from build123d import *

# Parameters (mm, degrees)
BOSS_EXTRUDE1_DEPTH = 3.175


with BuildPart() as part:
    # Sketch1 → Boss-Extrude1 (new body)
    with BuildSketch(Plane(origin=(0, 0, 0), x_dir=(1, 0, 0), z_dir=(0, 1, 0))):
        Polygon((0, -25.4), (0, 25.4), (25.4, 25.4), (25.4, 28.575), (114.3, 28.575), (114.3, 25.4), (139.7, 25.4), (165.1, 25.4), (165.1, 28.575), (254, 28.575), (254, 25.4), (279.4, 25.4), (304.8, 25.4), (304.8, 28.575), (393.7, 28.575), (393.7, 25.4), (419.1, 25.4), (444.5, 25.4), (444.5, 28.575), (533.4, 28.575), (533.4, 25.4), (558.8, 25.4), (558.8, -25.4), (533.4, -25.4), (533.4, -28.575), (444.5, -28.575), (444.5, -25.4), (419.1, -25.4), (393.7, -25.4), (393.7, -28.575), (304.8, -28.575), (304.8, -25.4), (279.4, -25.4), (254, -25.4), (254, -28.575), (165.1, -28.575), (165.1, -25.4), (139.7, -25.4), (114.3, -25.4), (114.3, -28.575), (25.4, -28.575), (25.4, -25.4), align=None)
    extrude(amount=BOSS_EXTRUDE1_DEPTH)


solid = part.part
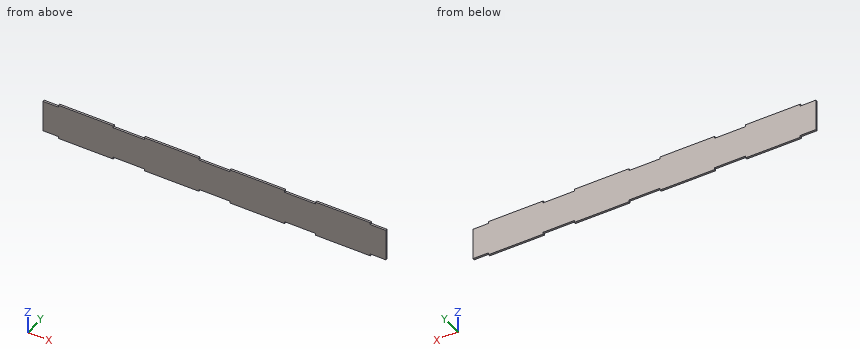
Read the model definition and answer for the solid it produces. Units are mm, in the model's axes. Coordinates: 2 decimals unless noted, no trailing zeros. Order: outer loops, then holes, each group sorted by start corner. A loop starts at its lowest first (then second) coordinate and runs counter-clockwise, first axis right, second up. Notation, with made-up numbers: (7.5, 3) -> (12.5, 3) arc R10 cw to (12.5, 9) -> close; hole circle Ø7 at (29, 38.25). An arc over 180 degrees is marked (long way). Answer as a JSON object with one key per item and string values.
1) Each of these flat-tipped pins is pushed along its axis until it touches: pin 1 (1.6 mm diameter, centred on y = 2, z = 26.5, fed in from -X); pin 2 (1 mm diameter, centred on x = 541, y = 1, fed in from +Z); pin 3 (1 mm diameter, centred on x = 291, y = 2.5, fed in from -Z). Where does it stop, or does it pass through?
Model answer:
{"pin 1": "stops at x = 25.4", "pin 2": "stops at z = 25.4", "pin 3": "stops at z = -25.4"}
2) Consider line 1 along X through (y, z) = (1.35, 26); line 2 along Z through (x, y) = (423, 0.4). Determine where each line is inside the solid, lowest interval first. Write a range as from..to.
Model answer:
{"line 1": "x = 25.4..114.3, 165.1..254, 304.8..393.7, 444.5..533.4", "line 2": "z = -25.4..25.4"}
3) A cutting plane is placed at A-A, the plane x = 150. Determine the outline of the cut face in (y, z) (3 decimals).
Model answer:
{"outline": "(0, -25.4) -> (3.175, -25.4) -> (3.175, 25.4) -> (0, 25.4) -> close"}
